Check sheet for the modelled part. Datum: model origin and axes. Units: mm. A direction names the side the tool comes from. Give positions to 0.01 mm unless a question says otherwise; leave off trailing zeros. Write each loop counter-clockwise with the first axis right and the second up, starting at its lowest first coordinate (ties: lowest second). Pieces come first, ordered by that corner, then holes. Notation, with made-up numbers: (14, 55.25) -> (42, 55.25) arc R25 ccw to (42, 73.25) -> close; hole circle Ø11 at (-32, 32.25). An arc over 180 degrees is marked (long way). Use a Markdown table: item, result. Add a question column.
1. Release check for a two-part mould opening along Z. For faces 1 (the cylindrical face through (-21.6, 0, -1.2)), 2 (the cylindrical face through (-0.312, -0.006, 20.005)), 3 (the flat face through (2.2, 16.4, -7.1)), 4 (the cylindrical face through (-20.234, -0.006, -6.735)) record: released by +Z, released by -Z, zero draft, split by the parting line, or undercut.
2. Scan lines: probe 1 along Z at (x, y) = (20, 0.1); probe 2 along Y at (x, z) = (18, 1.5); probe 3 along X at (y, z) = (6.25, -5). Record each from-to range of solid material in increasing order. Write a range as [from, to].
3. Cross-section at B-B (x = 20). Enter the section's corners in (y, z).
4. Cross-section at C-C (x = 0). Enter the section's corners in (y, z).
5. Set-up check for faces 5 (the cylindrical face through (18.4, 0, -1.2)), 6 (the flat face through (0, 0.4, -14)): record each of +Z, -Z, +X, -X, +Y, -Y from which the full face is reachable in a straight line by a thin tool's end or side.
6. Gauge pin test, flat ends, axial feed: P1, Ø6, axis at x = -3.5, z = 8.5, coming from the +Y side; P2, Ø3, axis at y = 7.5, z = 13.5, coming from the +X side; P3, Ø10, axis at x = -13, y = 4.5, coming from the -Z side. Record the tip position at first contact, or that the pin passes through.
7. Cross-section at D-D (y = 11.25). Enter the section's corners in (x, z).
8. Cross-section at A-A (z = 0). Enter the section's corners in (x, y), then the cut area to 3 significant figures.
from build123d import *
from build123d.topology import SkipClean

# Parameters (mm, degrees)
FILLET_1_R          = 3
SKETCH_2_R          = 2
CUT_EXTRUDE_1_DEPTH = 10


with BuildPart() as part:
    # Sketch 1 → Revolve 1 (revolve)
    with BuildSketch(Plane.XY):
        Polygon((0, -0.4), (0, 16.4), (-6.979971347, 16.4), (-6.979971347, 16.177681197), (-7.205553414, 16.177681197), (-7.205553414, 16.4), (-13.5, 16.4), (-13.5, 0.4), (-24.5, 0.4), (-24.5, -0.4), align=None)
    revolve(axis=Axis((0, 20.6, 0), (0, -1, 0)))

    # Sketch 1_3 → Revolve 2 (revolve)
    with SkipClean():  # the faces are left unmerged after this step: merging them gives an invalid solid
        with BuildSketch(Plane.XY):
            with BuildLine():
                Line((0, 16.4), (6.979971347, 16.4))
                ThreePointArc((6.979971347, 16.4), (4.073082371, 19.4690472), (0, 20.6))
                Line((0, 20.6), (0, 16.4))
            make_face()
            with BuildLine():
                Line((-6.979971347, 16.4), (0, 16.4))
                Line((0, 16.4), (0, 20.6))
                ThreePointArc((0, 20.6), (-4.073082371, 19.4690472), (-6.979971347, 16.4))
            make_face()
        revolve(axis=Axis((0, 20.6, 0), (0, -1, 0)))
    add(part.part.scale(1), mode=Mode.REPLACE)  # the faces are merged on a copy

    # Fillet 1
    fillet_1_edges = [part.edges().sort_by_distance(p)[0] for p in [
        (13.5, 16.4, 0),
    ]]
    fillet(fillet_1_edges, radius=FILLET_1_R)

    # Sketch 2 → Cut-Extrude 1 (cut)
    with BuildSketch(Plane.XZ.offset(0.4)):
        with Locations((-20, 0)):
            Circle(SKETCH_2_R)
        with Locations((20, 0)):
            Circle(SKETCH_2_R)
        with BuildLine():
            ThreePointArc((-24.25, -3.491060011), (0, -24.5), (24.25, -3.491060011))
            ThreePointArc((24.25, -3.491060011), (23.568060584, -4.185563721), (22.77437579, -4.748982941))
            ThreePointArc((22.77437579, -4.748982941), (20.265276607, -6.702825437), (18.357504114, -9.24712953))
            ThreePointArc((18.357504114, -9.24712953), (0, -20.006865782), (-18.357504114, -9.24712953))
            ThreePointArc((-18.357504114, -9.24712953), (-20.265276607, -6.702825437), (-22.77437579, -4.748982941))
            ThreePointArc((-22.77437579, -4.748982941), (-23.568060584, -4.185563721), (-24.25, -3.491060011))
        make_face()
        with BuildLine():
            ThreePointArc((22.77437579, 4.748982941), (23.568060584, 4.185563721), (24.25, 3.491060011))
            ThreePointArc((24.25, 3.491060011), (0, 24.5), (-24.25, 3.491060011))
            ThreePointArc((-24.25, 3.491060011), (-23.568060584, 4.185563721), (-22.77437579, 4.748982941))
            ThreePointArc((-22.77437579, 4.748982941), (-20.265276607, 6.702825437), (-18.357504114, 9.24712953))
            ThreePointArc((-18.357504114, 9.24712953), (0, 20.006865782), (18.357504114, 9.24712953))
            ThreePointArc((18.357504114, 9.24712953), (20.265276607, 6.702825437), (22.77437579, 4.748982941))
        make_face()
    extrude(amount=-CUT_EXTRUDE_1_DEPTH, mode=Mode.SUBTRACT)


solid = part.part
Worked answers:
| question | item | result |
|---|---|---|
| 1 | face 1 | undercut |
| 1 | face 2 | released by +Z |
| 1 | face 3 | zero draft |
| 1 | face 4 | released by -Z |
| 2 | probe 1 | z = [-6.98, -2], [2, 6.98] |
| 2 | probe 2 | y = [-0.4, 0.4] |
| 2 | probe 3 | x = [-12.54, 12.54] |
| 3 | outline | (-0.4, -6.98) -> (0.4, -6.98) -> (0.4, -2) -> (-0.4, -2) -> close; (-0.4, 2) -> (0.4, 2) -> (0.4, 6.98) -> (-0.4, 6.98) -> close |
| 4 | outline | (-0.4, -20.01) -> (0.4, -20.01) -> (0.4, -13.5) -> (13.4, -13.5) arc R3 ccw to (16.4, -10.5) -> (16.4, -7.21) -> (16.18, -7.21) -> (16.18, -6.98) -> (16.4, -6.98) arc R7.9 ccw to (16.4, 6.98) -> (16.18, 6.98) -> (16.18, 7.21) -> (16.4, 7.21) -> (16.4, 10.5) arc R3 ccw to (13.4, 13.5) -> (0.4, 13.5) -> (0.4, 20.01) -> (-0.4, 20.01) -> close |
| 5 | face 5 | +Y, -Y |
| 5 | face 6 | +Y |
| 6 | P1 | stops at y = 17.61 |
| 6 | P2 | stops at x = 6.18 |
| 6 | P3 | stops at z = -17.4 |
| 7 | outline | circle Ø27 at (0, 0) |
| 8 | outline | (-24.5, -0.4) -> (-22, -0.4) -> (-22, 0.4) -> (-24.5, 0.4) -> close; (-18, -0.4) -> (18, -0.4) -> (18, 0.4) -> (13.5, 0.4) -> (13.5, 13.4) arc R3 ccw to (10.5, 16.4) -> (7.21, 16.4) -> (7.21, 16.18) -> (6.98, 16.18) -> (6.98, 16.4) arc R7.9 ccw to (-6.98, 16.4) -> (-6.98, 16.18) -> (-7.21, 16.18) -> (-7.21, 16.4) -> (-10.5, 16.4) arc R3 ccw to (-13.5, 13.4) -> (-13.5, 0.4) -> (-18, 0.4) -> close; (22, -0.4) -> (24.5, -0.4) -> (24.5, 0.4) -> (22, 0.4) -> close |
| 8 | area | 503 mm² |
